For this review, take the finished solid that the model builds, in its own axes (mm). A direction names the side the tool comes from. Coordinates: 2 decimals unless noted, no trailing zeros. Write each loop counter-clockwise with the first axis right and the second up, starting at its lowest first coordinate (ties: lowest second). Pieces come first, ordered by that corner, then holes. Notation, with made-up numbers: (-35.75, 8) -> (14.25, 8) arc R26 ccw to (14.25, 23) -> close; hole circle Ø4 at (-6, 23). An arc over 180 degrees is marked (long way). One line per item, written item: value. Start each with the question number.
1) For probe 1 along X at (y, z) = (27.15, -11); probe 2 along X at (y, z) = (20.5, 4.5); probe 3 along X at (y, z) = (-17, 10), list the stretches that pass through material, from the lowest coordinate up. Write a range as from..to.
2) Add section B-B (y = -7). State the section outline as (x, z) points.
3) Mouldability with a two-part tool opening along Z and no side actions: class faces 6 (the flat face through (-33, 1, 0)), 7 (the cylindrical face through (-39.822, -22.546, 9.062)), 8 (the flat face through (24.414, 27, 22)), 9 (the cylindrical face through (46.42, -17.55, 9.82)) as released by +Z, released by -Z, zero draft, split by the parting line, or undercut.
4) Add section A-A (z = 16). State the section outline as (x, y) points, and give its area (3 significant figures).
5) Add section D-D (x = 35.5). State the section outline as (y, z) points, and give its area (3 significant figures).
6) Add section C-C (z = 10). State how many separate pieces and enclosed holes the cut face has, and give its area (3 significant figures).
7) For pin 1 Ø5 at (x, y) = (-32, 14) entering from +Z; pin 2 Ø6 at (y, z) = (-8.5, 1.5) entering from -X; pin 3 Ø3 at (x, z) = (-40.5, 11.5) entering from +Y, all flat-tipped, find the tip position at first contact; note any pin that passes through.
8) Machinability: for faces 1 (the flat face through (-15.586, 27, -8)), 2 (the flat face through (24.414, 27, -8)), 3 (the flat face through (42.414, 9, 10)), 4 (the flat face through (42, 1, 20)), 5 (the flat face through (-33.586, 9, 10)), which of the approach directions +Z, -Z, +X, -X, +Y, -Y give a long, thin tool a straight path to every point of the face, cutting with its end or side? Answer none if there is none.
from build123d import *

# Parameters (mm, degrees)
EXTRUDE_1_DEPTH     = 20
SKETCH_2_W          = 40
SKETCH_2_H          = 40
EXTRUDE_3_DEPTH     = 3
SKETCH_3_R          = 19
CUT_EXTRUDE_1_DEPTH = 3
SKETCH_4_R          = 1.25
CUT_EXTRUDE_2_DEPTH = 3
SKETCH_5_R          = 19
EXTRUDE_4_DEPTH     = 2
SKETCH_6_R          = 1.25
CUT_EXTRUDE_3_DEPTH = 2
EXTRUDE_5_DEPTH     = 20
CUT_EXTRUDE_4_DEPTH = 59
SKETCH_11_R         = 2.45
CUT_EXTRUDE_5_DEPTH = 59
SKETCH_12_R         = 4.5
CUT_EXTRUDE_6_DEPTH = 59
CHAMFER_1_SIZE      = 1


with BuildPart() as part:
    # 草图1 → 凸台-拉伸1 (new body)
    with BuildSketch(Plane.XY):
        Polygon((-33.585585586, 27.988738739), (-33.585585586, -25.011261261), (-30.585585586, -25.011261261), (-30.585585586, 24.988738739), (39.414414414, 24.988738739), (39.414414414, -25.011261261), (42.414414414, -25.011261261), (42.414414414, 27.988738739), align=None)
    extrude(amount=EXTRUDE_1_DEPTH)

    # 草图2 → 凸台-拉伸3 (add)
    with BuildSketch(Plane(origin=(0, 27.988738739, 0), x_dir=(1, 0, 0), z_dir=(0, 1, 0))):
        with Locations((4.414414414, -5)):
            Rectangle(SKETCH_2_W, SKETCH_2_H)
    extrude(amount=-EXTRUDE_3_DEPTH)

    # 草图3 → 切除-拉伸1 (cut)
    with BuildSketch(Plane(origin=(0, 27.988738739, 0), x_dir=(1, 0, 0), z_dir=(0, 1, 0))):
        with Locations((4.414414414, -5)):
            Circle(SKETCH_3_R)
    extrude(amount=-CUT_EXTRUDE_1_DEPTH, mode=Mode.SUBTRACT)

    # 草图4 → 切除-拉伸2 (cut)
    with BuildSketch(Plane(origin=(0, 27.988738739, 0), x_dir=(1, 0, 0), z_dir=(0, 1, 0))):
        with Locations((20.414414414, 11)):
            Circle(SKETCH_4_R)
        with Locations((20.414414414, -21)):
            Circle(SKETCH_4_R)
        with Locations((-11.585585586, -21)):
            Circle(SKETCH_4_R)
        with Locations((-11.585585586, 11)):
            Circle(SKETCH_4_R)
    extrude(amount=-CUT_EXTRUDE_2_DEPTH, mode=Mode.SUBTRACT)

    # 草图5 → 凸台-拉伸4 (add)
    with BuildSketch(Plane(origin=(0, 27.988738739, 0), x_dir=(1, 0, 0), z_dir=(0, 1, 0))):
        Polygon((-33.585585586, -20), (-15.585585586, -20), (-15.585585586, -25), (24.414414414, -25), (24.414414414, -20), (42.414414414, -20), (42.414414414, 0), (24.414414414, 0), (24.414414414, 15), (-15.585585586, 15), (-15.585585586, 0), (-33.585585586, 0), align=None)
        with Locations((4.414414414, -5)):
            Circle(SKETCH_5_R, mode=Mode.SUBTRACT)
    extrude(amount=EXTRUDE_4_DEPTH)

    # 草图6 → 切除-拉伸3 (cut)
    with BuildSketch(Plane.XZ.offset(-27.988738739)):
        with Locations((20.414414414, 21)):
            Circle(SKETCH_6_R)
        with Locations((20.414414414, -11)):
            Circle(SKETCH_6_R)
        with Locations((-11.585585586, -11)):
            Circle(SKETCH_6_R)
        with Locations((-11.585585586, 21)):
            Circle(SKETCH_6_R)
    extrude(amount=-CUT_EXTRUDE_3_DEPTH, mode=Mode.SUBTRACT)

    # 草图7 → 凸台-拉伸5 (add)
    with BuildSketch(Plane(origin=(0, 0, 0), x_dir=(-1, 0, 0), z_dir=(0, 0, -1))):
        Polygon((33.585585586, -25.011261261), (53.585585586, -25.011261261), (33.585585586, -11.021791252), align=None)
    extrude(amount=-EXTRUDE_5_DEPTH)

    # 草图10 → 切除-拉伸4 (cut)
    with BuildSketch(Plane(origin=(0, 0, -15), x_dir=(-1, 0, 0), z_dir=(0, 0, -1))):
        Polygon((-4.414414414, 24.988738739), (-4.414414414, -56.650285004), (-57.489425736, -56.650285004), (-57.489425736, 45.664413948), (-4.414414414, 45.664413948), align=None)
    extrude(amount=-CUT_EXTRUDE_4_DEPTH, mode=Mode.SUBTRACT)

    # 草图11 → 切除-拉伸5 (cut)
    with BuildSketch(Plane.XZ.offset(25.011261261)):
        with Locations((-42.085585586, 10)):
            Circle(SKETCH_11_R)
    extrude(amount=-CUT_EXTRUDE_5_DEPTH, mode=Mode.SUBTRACT)

    # 草图12 → 切除-拉伸6 (cut)
    with BuildSketch(Plane(origin=(0, -20.011261261, 0), x_dir=(-1, 0, 0), z_dir=(0, -1, 0))):
        with Locations((42.085585586, -10)):
            Circle(SKETCH_12_R)
    extrude(amount=-CUT_EXTRUDE_6_DEPTH, mode=Mode.SUBTRACT)

    # 镜向2: part across plane


with BuildPart() as part_1:
    add(part.part)
    add(part.part.mirror(Plane(origin=(4.414414414, 24.988738739, 44), x_dir=(0, 0, 1), z_dir=(-1, 0, 0))))

    # 倒角1
    chamfer_1_edges = [part_1.edges().sort_by_distance(p)[0] for p in [
        (42.414414414, 29.988738739, 10),
        (-33.585585586, 29.988738739, 10),
    ]]
    chamfer(chamfer_1_edges, length=CHAMFER_1_SIZE)


solid = part_1.part
Numbers:
1. probe 1: -15.59..-12.84, -10.34..-5.83, 14.66..19.16, 21.66..24.41
1. probe 2: -33.59..-30.59, 39.41..42.41
1. probe 3: -37.59..-30.59, 39.41..46.41
2. outline: (-33.59, 0) -> (-30.59, 0) -> (-30.59, 20) -> (-33.59, 20) -> close; (39.41, 0) -> (42.41, 0) -> (42.41, 20) -> (39.41, 20) -> close
3. face 6: released by -Z
3. face 7: undercut
3. face 8: zero draft
3. face 9: undercut
4. outline: (-53.59, -25.01) -> (-30.59, -25.01) -> (-30.59, 24.99) -> (-11.08, 24.99) -> (-11.08, 29.99) -> (-32.59, 29.99) -> (-33.59, 28.99) -> (-33.59, -11.02) -> close; (19.91, 24.99) -> (39.41, 24.99) -> (39.41, -25.01) -> (62.41, -25.01) -> (42.41, -11.02) -> (42.41, 28.99) -> (41.41, 29.99) -> (19.91, 29.99) -> close
4. area: 804 mm²
5. outline: (24.99, 0) -> (29.99, 0) -> (29.99, 20) -> (24.99, 20) -> close
5. area: 100 mm²
6. separate pieces: 4
6. enclosed holes: 0
6. area: 672 mm²
7. pin 1: z = 20
7. pin 2: x = -34.27
7. pin 3: y = -20.01
8. face 1: -Z, -X, +Y, -Y
8. face 2: -Z, +X, +Y, -Y
8. face 3: +Z, -Z, +X, +Y
8. face 4: +Z, +X, +Y, -Y
8. face 5: +Z, -Z, -X, +Y
